Input: part model. Units: mm. Frame: model coordinates. A direction names the side the tool comes from. Coordinates: 2 decimals unless noted, no trailing zeros. Loops run counter-clockwise (first coordinate to the right, second up) from the corner with the lowest first, then second, coordinate; pieces in that order, holes last.
(1) Section D-D, the plane x = -5.25. Return loops of the section in (y, z), then the cut area to 3 significant figures.
(2) Set-up query: faces 4 (the face through (6, 5, -2)), 5 (the face through (1.802, 3.521, 5.723)). Return all of +Z, -Z, +X, -X, +Y, -Y with unobstructed straight access to the full face (end or side cutting, diameter ignored); none if empty.
(3) Section C-C, the plane y = 3.3. Return loops of the section in (x, z).
(4) Section A-A, the plane x = 0. Return loops of the section in (y, z).
(5) Line query: L1, parallel to X at y = 4.35, z = 0; L2, parallel to X at y = 0.6, z = 0; L3, parallel to Z at x = 0.25, y = 2.25. Output: solid intervals per line, ascending.
(6) Contact query for flat-ended pins moving along their axis: P1, Ø9.5, axis at x = 0, z = 0, coming from the -Y side; P2, Ø3, axis at y = 2, z = 6.5, coming from the +X side (3 decimals); P3, Ø1.5, axis at x = -0.5, z = 0.5, coming from the -Y side; P4, Ø6, axis at x = -0.5, z = -2.5, coming from the +Y side. Output: stop coordinate, or through.
(7) Mould query, pull axis Z, two halves, no side actions, for faces 1 (the face through (0.9, 1.01, 2.86)), 2 (the face through (0.1, 0, 3.4)), 3 (the face through (-7.81, 2.46, -1.73)). Classes: released by +Z, released by -Z, zero draft, split by the parting line, or undercut.
(8) Section B-B, the plane z = 0. Return loops of the section in (x, y), then the cut area to 3 significant figures.
```python
from build123d import *

# Parameters (mm, degrees)
SKETCH_1_R          = 8
EXTRUDE_1_DEPTH     = 5
SKETCH_2_R          = 6
CUT_EXTRUDE_1_DEPTH = 3
SKETCH_3_R          = 3
CUT_EXTRUDE_2_DEPTH = 12.704699911


with BuildPart() as part:
    # 草图1 → 凸台-拉伸1 (new body)
    with BuildSketch(Plane(origin=(0, 0, 0), x_dir=(1, 0, 0), z_dir=(0, 1, 0))):
        with Locations(Location((0, 0, 0), (0, 0, 270))):
            Circle(SKETCH_1_R)
    extrude(amount=EXTRUDE_1_DEPTH)

    # 草图2 → 切除-拉伸1 (cut)
    with BuildSketch(Plane(origin=(0, 5, 0), x_dir=(1, 0, 0), z_dir=(0, 1, 0))):
        with Locations(Location((0, 0, 0), (0, 0, 270))):
            Circle(SKETCH_2_R)
    extrude(amount=-CUT_EXTRUDE_1_DEPTH, mode=Mode.SUBTRACT)

    # 草图3 → 切除-拉伸2 (cut, through all)
    with BuildSketch(Plane(origin=(0, 2, 0), x_dir=(1, 0, 0), z_dir=(0, 1, 0))):
        with Locations(Location((0, 0, 0), (0, 0, 270))):
            Circle(SKETCH_3_R)
    extrude(amount=-CUT_EXTRUDE_2_DEPTH, mode=Mode.SUBTRACT)


solid = part.part
```
Report:
1. outline: (0, -6.04) - (5, -6.04) - (5, -2.9) - (2, -2.9) - (2, 2.9) - (5, 2.9) - (5, 6.04) - (0, 6.04) - close
1. area: 42.9 mm2
2. face 4: +Z, -Z, +X, -X, +Y
2. face 5: +Y
3. outline: circle Ø16 at (0, 0); hole circle Ø12 at (0, 0)
4. outline: (0, -8) - (5, -8) - (5, -6) - (2, -6) - (2, -3) - (0, -3) - close; (0, 3) - (2, 3) - (2, 6) - (5, 6) - (5, 8) - (0, 8) - close
5. L1: x = -8 to -6, 6 to 8
5. L2: x = -8 to -3, 3 to 8
5. L3: z = -8 to -5.99, 5.99 to 8
6. P1: stops at y = 0
6. P2: stops at x = 6.245
6. P3: passes through
6. P4: stops at y = 2
7. face 1: undercut
7. face 2: zero draft
7. face 3: split by the parting line
8. outline: (-8, 0) - (-3, 0) - (-3, 2) - (-6, 2) - (-6, 5) - (-8, 5) - close; (3, 0) - (8, 0) - (8, 5) - (6, 5) - (6, 2) - (3, 2) - close
8. area: 32.0 mm2
